from build123d import *

# Parameters (mm, degrees)
SKETCH_1_W               = 1
SKETCH_1_H               = 12
SKETCH_1_W_2             = 1.5
SKETCH_1_R               = 6
SKETCH_1_R_2             = 5
EXTRUDE_1_DEPTH          = 3.5
CUT_EXTRUDE_1_DEPTH      = 17.324827717
CUT_EXTRUDE_1_DEPTH_BACK = 17.324827717
SKETCH_2_R               = 0.75
SKETCH_2_R_2             = 0.5
SKETCH_3_R               = 0.75
SKETCH_3_R_2             = 0.5
CUT_EXTRUDE_2_DEPTH      = 3.5


with BuildPart() as part:
    # Эскиз1 → Бобышка-Вытянуть1 (new body)
    # profile 1 of 7: a face of its own
    with BuildSketch(Plane(origin=(0, 0, 0), x_dir=(1, 0, 0), z_dir=(0, 1, 0))):
        with Locations((-10, 0)):
            Rectangle(SKETCH_1_W, SKETCH_1_H)
    # profile 2 of 7: a face of its own
    with BuildSketch(Plane(origin=(0, 0, 0), x_dir=(1, 0, 0), z_dir=(0, 1, 0))):
        with Locations((-8.75, 0)):
            Rectangle(SKETCH_1_W_2, SKETCH_1_H)
    # profile 3 of 7: a face of its own
    with BuildSketch(Plane(origin=(0, 0, 0), x_dir=(1, 0, 0), z_dir=(0, 1, 0))):
        with Locations((-7.5, 0)):
            Rectangle(SKETCH_1_W, SKETCH_1_H)
    # profile 4 of 7: a face of its own
    with BuildSketch(Plane(origin=(0, 0, 0), x_dir=(1, 0, 0), z_dir=(0, 1, 0))):
        with Locations((-6.5, 0)):
            Rectangle(SKETCH_1_W, SKETCH_1_H)
    # profile 5 of 7: a face of its own
    with BuildSketch(Plane(origin=(0, 0, 0), x_dir=(1, 0, 0), z_dir=(0, 1, 0))):
        with BuildLine():
            Line((-6, -5e-09), (-6, -6))
            Line((-6, -6), (0, -6))
            ThreePointArc((0, -6), (-4.242640685, -4.242640689), (-6, -5e-09))
        make_face()
    # profile 6 of 7: a face of its own
    with BuildSketch(Plane(origin=(0, 0, 0), x_dir=(1, 0, 0), z_dir=(0, 1, 0))):
        Circle(SKETCH_1_R)
        with Locations(Location((0, 0, 0), (0, 0, 270))):
            Circle(SKETCH_1_R_2, mode=Mode.SUBTRACT)
    # profile 7 of 7: a face of its own
    with BuildSketch(Plane(origin=(0, 0, 0), x_dir=(1, 0, 0), z_dir=(0, 1, 0))):
        with BuildLine():
            Line((-6, 6), (-6, -5e-09))
            ThreePointArc((-6, -5e-09), (-4.242640689, 4.242640685), (0, 6))
            Line((0, 6), (-6, 6))
        make_face()
    extrude(amount=EXTRUDE_1_DEPTH)

    # Эскиз2 → Вырез-Вытянуть1 (cut, two sides: drawn at the far end of the back side and taken through both)
    with BuildSketch(Plane.XY.offset(6).offset(-CUT_EXTRUDE_1_DEPTH_BACK)):
        with Locations((-8.75, 1.75)):
            Circle(SKETCH_2_R)
        with Locations((-6.5, 1.75)):
            Circle(SKETCH_2_R_2)
    extrude(amount=CUT_EXTRUDE_1_DEPTH + CUT_EXTRUDE_1_DEPTH_BACK, mode=Mode.SUBTRACT)

    # Эскиз3 → Вырез-Вытянуть2 (cut)
    with BuildSketch(Plane(origin=(0, 3.5, 0), x_dir=(1, 0, 0), z_dir=(0, 1, 0))):
        with Locations(Location((-4.767766953, 4.767766953, 0), (0, 0, 270))):
            Circle(SKETCH_3_R)
        with Locations(Location((-4.767766953, -4.767766953, 0), (0, 0, 90))):
            Circle(SKETCH_3_R_2)
    extrude(amount=-CUT_EXTRUDE_2_DEPTH, mode=Mode.SUBTRACT)


solid = part.part
Verification items for the finished model (mm, model axes). Coordinates: 2 decimals unless noted, no trailing zeros. Order: outer loops, then holes, each group sorted by start corner. A loop starts at its lowest first (then second) coordinate and runs counter-clockwise, first axis right, second up. Notation, with made-up numbers: (8.5, -35) -> (34.5, -35) arc R15 cw to (34.5, -12) -> close; hole circle Ø2 at (66.5, -25.75). An arc over 180 degrees is marked (long way). Put each result on its own line as item: value. Start each with the question number.
1. Cross-section at C-C, the plane y = 2. Record the boundary of the cut face in (x, z).
2. Mould release check, pull along Z, two halves, no side actions. Record for faces 1 (the cylindrical face through (6, 2, 0)), 2 (the cylindrical face through (-6.023, 1.9, -0.084)), 3 (the cylindrical face through (-4.576, 1.774, 4.306)), 4 (the flat face through (-5, 2, 6)): released by +Z, released by -Z, zero draft, split by the parting line, or undercut.
3. Cross-section at D-D, the plane z = -2.75. Record the boundary of the cut face in (x, y).
4. Go/stop test with flat-tipped pins: pin 1 Ø1.5 at (x, y) = (2, 2) entering from +Z; pin 2 Ø0.9 at (x, y) = (-8.75, 1.75) entering from -Z. Record where each tip stops, or that it passes through.
5. Cross-section at B-B, the plane z = 0. Record the boundary of the cut face in (x, y), then the cut area to 3 significant figures.
6. Cross-section at A-A, the plane x = -8.75. Record the boundary of the cut face in (y, z), then the cut area to 3 significant figures.
7. Material ranges on L1, parallel to Y at x = -8.75, z = 2; L2, parallel to X at y = 2, z = 1.5; L3, parallel to X at y = 0.3, z = 0, recorded low to high. Write a range as [from, to].
Computed:
1. outline: (-10.5, -6) -> (-9.46, -6) -> (-9.46, 6) -> (-10.5, 6) -> close; (-8.04, -6) -> (-6.93, -6) -> (-6.93, 6) -> (-8.04, 6) -> close; (-6.07, -6) -> (0, -6) arc R6 ccw to (0, 6) -> (-6.07, 6) -> close; hole circle Ø1.5 at (-4.77, -4.77); hole circle Ø1 at (-4.77, 4.77); hole circle Ø10 at (0, 0)
2. face 1: split by the parting line
2. face 2: zero draft
2. face 3: undercut
2. face 4: released by +Z
3. outline: (-10.5, 0) -> (-4.18, 0) -> (-4.18, 3.5) -> (-10.5, 3.5) -> close; (4.18, 0) -> (5.33, 0) -> (5.33, 3.5) -> (4.18, 3.5) -> close; hole circle Ø1.5 at (-8.75, 1.75); hole circle Ø1 at (-6.5, 1.75)
4. pin 1: z = 5.87
4. pin 2: through
5. outline: (-10.5, 0) -> (-5, 0) -> (-5, 3.5) -> (-10.5, 3.5) -> close; (5, 0) -> (6, 0) -> (6, 3.5) -> (5, 3.5) -> close; hole circle Ø1.5 at (-8.75, 1.75); hole circle Ø1 at (-6.5, 1.75)
5. area: 20.2 mm2
6. outline: (0, -6) -> (1, -6) -> (1, 6) -> (0, 6) -> close; (2.5, -6) -> (3.5, -6) -> (3.5, 6) -> (2.5, 6) -> close
6. area: 24.0 mm2
7. L1: [0, 1], [2.5, 3.5]
7. L2: [-10.5, -9.46], [-8.04, -6.93], [-6.07, -4.77], [4.77, 5.81]
7. L3: [-10.5, -5], [5, 6]
